Source: CAD feature listing. Evaluate the final solid. Frame: model axes, mm. A direction names the side the tool comes from. Round coordinates to 2 decimals unless told otherwise and drop trailing zeros. Order: outer loops, then holes, each group sorted by start corner. A loop starts at its lowest first (then second) coordinate and runs counter-clockwise, first axis right, second up. Notation, with made-up numbers: (-13, 21) -> (44, 21) arc R15 ccw to (44, 39) -> close; hole circle Ø9 at (61.25, -3). An arc over 180 degrees is marked (long way). Write item = value, one per line. Start each with the question number.
(1) Ray query, line 1 (X direction, y = 6.9, z = 0) (3 decimals); line 2 (X direction, y = 4.5, z = 1.5); line 3 (Y direction, x = 24, z = -2.25) (1 decimal). Return the intervals inside material, ascending.
(2) Cut plane C-C on z = 0. Give the number of separate pieces and of enclosed holes in the cut face, then the cut area to 3 significant figures.
(3) Cut plane A-A on x = -4. Return the cut outline in (y, z) (1 decimal), then the cut area to 3 significant figures.
(4) Cut plane B-B on y = -7.5. Return the cut outline in (x, z) (3 decimals).
(5) Draft query along X for faces 5 (the face through (25, 5.398, 0)), 6 (the face through (-14.729, 0.076, -3.994)), 7 (the face through (2.03, 7.43, -1.05)), 8 (the face through (15.875, 0, 0)). Return one class per face: released by +X, released by -X, zero draft, split by the parting line, or undercut.
(6) Contact query for flat-ended pins moving along their axis: pin 1 Ø1.3 at (y, z) = (-0.5, 0) entering from +X (3 decimals); pin 2 Ø3 at (y, z) = (-0.5, -0.5) entering from -X (3 decimals); pin 3 Ø1 at (y, z) = (-6.5, 2.5) entering from +X. Output: stop coordinate, or through.
(7) Reachability of faces 1 (the face through (-38.734, 7.49, 0.112)), 2 (the face through (32, 7, -2.286)), 3 (the face through (-9.401, 0.076, -3.994)), 4 (the face through (-9.401, 0.076, 3.994)) from +Z, -Z, +X, -X, +Y, -Y: full face, straight path, thin tool, end or side. Return the list, or none.
(8) Cut plane D-D on x = 14. Return the cut outline in (y, z) (1 decimal).
from build123d import *

# Parameters (mm, degrees)
SKETCH1_R           = 2.286
BOSS_EXTRUDE1_DEPTH = 9.525
SKETCH3_W           = 22.86
SKETCH3_H           = 10.795
SKETCH3_W_2         = 16.51
CUT_EXTRUDE1_DEPTH  = 42.162500531
FILLET1_R           = 3.81


with BuildPart() as part:
    # Sketch1 → Boss-Extrude1 (new, symmetric)
    with BuildSketch(Plane(origin=(0, 0, 0), x_dir=(1, 0, 0), z_dir=(0, 1, 0))):
        with BuildLine():
            Line((33.655, -5.08), (-33.655, -5.08))
            ThreePointArc((-33.655, -5.08), (-38.735, 0), (-33.655, 5.08))
            Line((-33.655, 5.08), (33.655, 5.08))
            ThreePointArc((33.655, 5.08), (38.735, 0), (33.655, -5.08))
        make_face()
        with Locations(Location((0, 0, 0), (0, 0, 90))):
            Circle(SKETCH1_R, mode=Mode.SUBTRACT)
        with BuildLine():
            Line((33.655, -2.286), (29.845, -2.286))
            ThreePointArc((29.845, -2.286), (27.559, 0), (29.845, 2.286))
            Line((29.845, 2.286), (33.655, 2.286))
            ThreePointArc((33.655, 2.286), (35.941, 0), (33.655, -2.286))
        make_face(mode=Mode.SUBTRACT)
        with BuildLine():
            Line((-33.655, 2.286), (-29.845, 2.286))
            ThreePointArc((-29.845, 2.286), (-27.559, 0), (-29.845, -2.286))
            Line((-29.845, -2.286), (-33.655, -2.286))
            ThreePointArc((-33.655, -2.286), (-35.941, 0), (-33.655, 2.286))
        make_face(mode=Mode.SUBTRACT)
    extrude(amount=BOSS_EXTRUDE1_DEPTH, both=True)

    # Sketch3 → Cut-Extrude1 (cut, through all)
    with BuildSketch(Plane.XY.offset(5.08)):
        with Locations((-27.305, 0)):
            Rectangle(SKETCH3_W, SKETCH3_H)
        Rectangle(SKETCH3_W_2, SKETCH3_H)
        with Locations((27.305, 0)):
            Rectangle(SKETCH3_W, SKETCH3_H)
    extrude(amount=-CUT_EXTRUDE1_DEPTH, mode=Mode.SUBTRACT)

    # Fillet1
    fillet1_edges = [part.edges().sort_by_distance(p)[0] for p in [
        (15.875, 0, -5.08),
        (15.875, 0, 5.08),
        (-15.875, 0, 5.08),
        (-15.875, 0, -5.08),
        (-8.255, 0, -5.08),
        (8.255, 0, -5.08),
        (-8.255, 0, 5.08),
        (8.255, 0, 5.08),
    ]]
    fillet(fillet1_edges, radius=FILLET1_R - 0.0001)  # a hair under: the kernel refuses the full size


solid = part.part
Evaluation:
q1.line_1 = -38.735 to -35.941, -27.559 to -2.286, 2.286 to 27.559, 35.941 to 38.735
q1.line_2 = -15.87 to -8.26, 8.26 to 15.87
q1.line_3 = -9.5 to -5.4, 5.4 to 9.5
q2.separate_pieces = 6
q2.enclosed_holes = 0
q2.area = 628 mm^2
q3.outline = (-9.5, -5.1) -> (-5.4, -5.1) -> (-5.4, 5.1) -> (-9.5, 5.1) -> close; (5.4, -5.1) -> (9.5, -5.1) -> (9.5, 5.1) -> (5.4, 5.1) -> close
q3.area = 83.9 mm^2
q4.outline = (-33.655, -5.08) -> (33.655, -5.08) arc R5.08 ccw to (33.655, 5.08) -> (-33.655, 5.08) arc R5.08 ccw to start; hole (-33.655, -2.286) -> (-29.845, -2.286) arc R2.286 ccw to (-29.845, 2.286) -> (-33.655, 2.286) arc R2.286 ccw to start; hole circle Ø4.572 at (0, 0); hole (29.845, -2.286) -> (33.655, -2.286) arc R2.286 ccw to (33.655, 2.286) -> (29.845, 2.286) arc R2.286 ccw to start
q5.face_5 = zero draft
q5.face_6 = released by -X
q5.face_7 = undercut
q5.face_8 = released by +X
q6.pin_1 = 15.875
q6.pin_2 = -15.875
q6.pin_3 = 38.32
q7.face_1 = -X, +Y, -Y
q7.face_2 = +Y, -Y
q7.face_3 = -Z
q7.face_4 = +Z
q8.outline = (-9.5, -5.1) -> (-5.4, -5.1) -> (-5.4, -4.6) -> (5.4, -4.6) -> (5.4, -5.1) -> (9.5, -5.1) -> (9.5, 5.1) -> (5.4, 5.1) -> (5.4, 4.6) -> (-5.4, 4.6) -> (-5.4, 5.1) -> (-9.5, 5.1) -> close
